Read the model definition and answer for the solid it produces. Units are mm, in the model's axes. A direction names the side the tool comes from. Coordinates: 2 decimals unless noted, no trailing zeros. Loops run counter-clockwise (first coordinate to the right, second up) from the corner with the lowest first, then second, coordinate; pieces in that order, holes last. Notation, with made-up numbers: (-39, -30.5) -> (-10, -30.5) arc R28 ccw to (-10, -7.5) -> close; hole circle Ø6 at (-3.5, -23.5). An arc over 180 degrees is marked (long way). One line per question, with ' | ' between items. Start each with the question number.
```python
from build123d import *

# Parameters (mm, degrees)
F1_DEPTH = 71.882
F0_R     = 2.2225
F2_DEPTH = 5.0038


with BuildPart() as f1:
    # F0 (on Right) → F1 (new body)
    with BuildSketch(Plane.YZ):
        with BuildLine():
            Line((-23.495, 19.304), (-25.528179, 19.304))
            Line((-25.528179, 19.304), (-28.194, 16.638179))
            Line((-28.194, 16.638179), (-28.194, -16.638179))
            Line((-28.194, -16.638179), (-25.528179, -19.304))
            Line((-25.528179, -19.304), (-23.495, -19.304))
            ThreePointArc((-23.495, -19.304), (-20.531515, -20.531515), (-19.304, -23.495))
            Line((-19.304, -23.495), (-19.304, -25.528179))
            Line((-19.304, -25.528179), (-16.638179, -28.194))
            Line((-16.638179, -28.194), (16.638179, -28.194))
            Line((16.638179, -28.194), (19.304, -25.528179))
            Line((19.304, -25.528179), (19.304, -23.495))
            ThreePointArc((19.304, -23.495), (20.531515, -20.531515), (23.495, -19.304))
            Line((23.495, -19.304), (25.528179, -19.304))
            Line((25.528179, -19.304), (28.194, -16.638179))
            Line((28.194, -16.638179), (28.194, 16.638179))
            Line((28.194, 16.638179), (25.528179, 19.304))
            Line((25.528179, 19.304), (23.495, 19.304))
            ThreePointArc((23.495, 19.304), (20.531515, 20.531515), (19.304, 23.495))
            Line((19.304, 23.495), (19.304, 25.528179))
            Line((19.304, 25.528179), (16.638179, 28.194))
            Line((16.638179, 28.194), (-16.638179, 28.194))
            Line((-16.638179, 28.194), (-19.304, 25.528179))
            Line((-19.304, 25.528179), (-19.304, 23.495))
            ThreePointArc((-19.304, 23.495), (-20.531515, 20.531515), (-23.495, 19.304))
        make_face()
    extrude(amount=F1_DEPTH)

    # F0 (on Right) → F2 (join)
    with BuildSketch(Plane.YZ):
        with BuildLine():
            Line((-28.194, 16.638179), (-25.528179, 19.304))
            Line((-25.528179, 19.304), (-23.495, 19.304))
            ThreePointArc((-23.495, 19.304), (-20.531515, 20.531515), (-19.304, 23.495))
            Line((-19.304, 23.495), (-19.304, 25.528179))
            Line((-19.304, 25.528179), (-16.638179, 28.194))
            Line((-16.638179, 28.194), (-23.495, 28.194))
            ThreePointArc((-23.495, 28.194), (-26.817695, 26.817695), (-28.194, 23.495))
            Line((-28.194, 23.495), (-28.194, 16.638179))
        make_face()
        with Locations((-23.495, 23.495)):
            Circle(F0_R, mode=Mode.SUBTRACT)
        with BuildLine():
            Line((-23.495, 19.304), (-25.528179, 19.304))
            Line((-25.528179, 19.304), (-28.194, 16.638179))
            Line((-28.194, 16.638179), (-28.194, -16.638179))
            Line((-28.194, -16.638179), (-25.528179, -19.304))
            Line((-25.528179, -19.304), (-23.495, -19.304))
            ThreePointArc((-23.495, -19.304), (-20.531515, -20.531515), (-19.304, -23.495))
            Line((-19.304, -23.495), (-19.304, -25.528179))
            Line((-19.304, -25.528179), (-16.638179, -28.194))
            Line((-16.638179, -28.194), (16.638179, -28.194))
            Line((16.638179, -28.194), (19.304, -25.528179))
            Line((19.304, -25.528179), (19.304, -23.495))
            ThreePointArc((19.304, -23.495), (20.531515, -20.531515), (23.495, -19.304))
            Line((23.495, -19.304), (25.528179, -19.304))
            Line((25.528179, -19.304), (28.194, -16.638179))
            Line((28.194, -16.638179), (28.194, 16.638179))
            Line((28.194, 16.638179), (25.528179, 19.304))
            Line((25.528179, 19.304), (23.495, 19.304))
            ThreePointArc((23.495, 19.304), (20.531515, 20.531515), (19.304, 23.495))
            Line((19.304, 23.495), (19.304, 25.528179))
            Line((19.304, 25.528179), (16.638179, 28.194))
            Line((16.638179, 28.194), (-16.638179, 28.194))
            Line((-16.638179, 28.194), (-19.304, 25.528179))
            Line((-19.304, 25.528179), (-19.304, 23.495))
            ThreePointArc((-19.304, 23.495), (-20.531515, 20.531515), (-23.495, 19.304))
        make_face()
        with BuildLine():
            Line((-25.528179, -19.304), (-28.194, -16.638179))
            Line((-28.194, -16.638179), (-28.194, -23.495))
            ThreePointArc((-28.194, -23.495), (-26.817695, -26.817695), (-23.495, -28.194))
            Line((-23.495, -28.194), (-16.638179, -28.194))
            Line((-16.638179, -28.194), (-19.304, -25.528179))
            Line((-19.304, -25.528179), (-19.304, -23.495))
            ThreePointArc((-19.304, -23.495), (-20.531515, -20.531515), (-23.495, -19.304))
            Line((-23.495, -19.304), (-25.528179, -19.304))
        make_face()
        with Locations((-23.495, -23.495)):
            Circle(F0_R, mode=Mode.SUBTRACT)
        with BuildLine():
            Line((23.495, 28.194), (16.638179, 28.194))
            Line((16.638179, 28.194), (19.304, 25.528179))
            Line((19.304, 25.528179), (19.304, 23.495))
            ThreePointArc((19.304, 23.495), (20.531515, 20.531515), (23.495, 19.304))
            Line((23.495, 19.304), (25.528179, 19.304))
            Line((25.528179, 19.304), (28.194, 16.638179))
            Line((28.194, 16.638179), (28.194, 23.495))
            ThreePointArc((28.194, 23.495), (26.817695, 26.817695), (23.495, 28.194))
        make_face()
        with Locations((23.495, 23.495)):
            Circle(F0_R, mode=Mode.SUBTRACT)
        with BuildLine():
            Line((19.304, -25.528179), (16.638179, -28.194))
            Line((16.638179, -28.194), (23.495, -28.194))
            ThreePointArc((23.495, -28.194), (26.817695, -26.817695), (28.194, -23.495))
            Line((28.194, -23.495), (28.194, -16.638179))
            Line((28.194, -16.638179), (25.528179, -19.304))
            Line((25.528179, -19.304), (23.495, -19.304))
            ThreePointArc((23.495, -19.304), (20.531515, -20.531515), (19.304, -23.495))
            Line((19.304, -23.495), (19.304, -25.528179))
        make_face()
        with Locations((23.495, -23.495)):
            Circle(F0_R, mode=Mode.SUBTRACT)
    extrude(amount=-F2_DEPTH)


solid = f1.part
```
(1) Determine the mould class of faces 1 (the cylindrical face through (-2.467, -25.715, 23.593)), 2 (the flat face through (35, -24, 19.304)), 3 (the flat face through (0, -24, -21)) for opening direction Z: +Z half, -Z half, draft (parallel to the pull), parting line (faces both ways), or undercut.
(2) A tool of negligible diameter and unlimited length cuts with its end or side. For faces 4 (the flat face through (35.44, 17.99, 26.84)), 5 (the flat face through (35.44, 17.95, -26.88)), 6 (the cylindrical face through (35.438, -20.564, -20.499)), from which of +Z, -Z, +X, -X, +Y, -Y can it reach the whole face along a straight path? Write none if from no direction.
(3) Each of these flat-tipped pins is pushed along its axis until it touches: pin 1 Ø7 at (y, z) = (-23.495, 23.495) entering from +X; pin 2 Ø1 at (x, z) = (42, -24.5) entering from -Y; pin 3 Ø1 at (x, y) = (46, 24.5) entering from +Z. Where does it stop, or does it pass through?
(4) Section A-A on x = 26 is taken. Write down the section's boundary in (y, z) (3 decimals).
(5) Section B-B on z = -18 is taken. Write down the section's boundary in (x, y), plus the area to 3 significant figures.
(6) Find the intervals of material crossed by probe 1 along Y at (x, z) = (60, 25); probe 2 along Y at (x, z) = (18, 18); probe 3 along Z at (x, y) = (13, 20), in increasing order. Write a range as from..to.
Working result:
1) face 1: undercut | face 2: +Z half | face 3: draft
2) face 4: +Z, +X, +Y | face 5: -Z, +X, +Y | face 6: -Z, +X, -Y
3) pin 1: stops at x = 0 | pin 2: stops at y = -19.3 | pin 3: stops at z = 19.3
4) outline: (-28.194, -16.638) -> (-25.528, -19.304) -> (-23.495, -19.304) arc R4.191 cw to (-19.304, -23.495) -> (-19.304, -25.528) -> (-16.638, -28.194) -> (16.638, -28.194) -> (19.304, -25.528) -> (19.304, -23.495) arc R4.191 cw to (23.495, -19.304) -> (25.528, -19.304) -> (28.194, -16.638) -> (28.194, 16.638) -> (25.528, 19.304) -> (23.495, 19.304) arc R4.191 cw to (19.304, 23.495) -> (19.304, 25.528) -> (16.638, 28.194) -> (-16.638, 28.194) -> (-19.304, 25.528) -> (-19.304, 23.495) arc R4.191 cw to (-23.495, 19.304) -> (-25.528, 19.304) -> (-28.194, 16.638) -> close
5) outline: (-5, -28.19) -> (0, -28.19) -> (0, -26.83) -> (71.88, -26.83) -> (71.88, 26.83) -> (0, 26.83) -> (0, 28.19) -> (-5, 28.19) -> close | area: 4,140 mm2
6) probe 1: y = -19.3..19.3 | probe 2: y = -26.83..26.83 | probe 3: z = -21.18..21.18
